```python
from build123d import *

# Parameters (mm, degrees)
SKETCH_R            = 2.95
PAD_DEPTH           = 1
SKETCH001_R         = 2.5
PAD001_DEPTH        = 7.7
FILLET_R            = 2.5
SKETCH002_W         = 0.7
SKETCH002_H         = 0.7
PAD002_DEPTH        = 0.5
SKETCH003_W         = 0.5
SKETCH003_H         = 0.5
PAD003_DEPTH        = 10.5
LINEARPATTERN_COUNT = 2
LINEARPATTERN_PITCH = 2.54


with BuildPart() as part:
    # Sketch → Pad (new body)
    with BuildSketch(Plane.XY):
        Circle(SKETCH_R)
    extrude(amount=PAD_DEPTH)

    # Sketch001 (on Face3 of Pad) → Pad001 (join)
    with BuildSketch(Plane.XY.offset(1)):
        Circle(SKETCH001_R)
    extrude(amount=PAD001_DEPTH)

    # Fillet
    fillet_edges = [part.edges().sort_by_distance(p)[0] for p in [
        (-2.5, 0, 8.7),
    ]]
    fillet(fillet_edges, radius=FILLET_R)

    # Sketch002 (on Face5 of Fillet) → Pad002 (join)
    with BuildSketch(Plane(origin=(0, 0, 0), x_dir=(1, 0, 0), z_dir=(0, 0, -1))):
        with Locations((-1.27, 0)):
            Rectangle(SKETCH002_W, SKETCH002_H)
    pad002 = extrude(amount=PAD002_DEPTH)

    # Sketch003 (on Face10 of Pad002) → Pad003 (join)
    with BuildSketch(Plane(origin=(0, 0, -0.5), x_dir=(1, 0, 0), z_dir=(0, 0, -1))):
        with Locations((-1.27, 0)):
            Rectangle(SKETCH003_W, SKETCH003_H)
    pad003 = extrude(amount=PAD003_DEPTH)

    # LinearPattern: Pad002, Pad003 ×2
    with Locations(*[(i * LINEARPATTERN_PITCH, 0, 0) for i in range(1, LINEARPATTERN_COUNT)]):
        add(pad002)
        add(pad003)


solid = part.part
```
Input: part model. Units: mm. Frame: model coordinates. A direction names the side the tool comes from. Coordinates: 2 decimals unless noted, no trailing zeros. Write each loop counter-clockwise with the first axis right and the second up, starting at its lowest first coordinate (ties: lowest second). Pieces come first, ordered by that corner, then holes. Notation, with made-up numbers: (84.5, -40) - (132.5, -40) arc R21 ccw to (132.5, -15) - close; hole circle Ø2 at (32.5, 83). An arc over 180 degrees is marked (long way). Put each result on its own line as item: value. Start each with the question number.
1) Reachability of faces 1 (the face through (-0.54, -2.44, 3.56)), 2 (the face through (-2.947, 0.13, 0.493)) from +Z, -Z, +X, -X, +Y, -Y: full face, straight path, thin tool, end or side. Return the list, or none.
2) Cut plane B-B (y = 0). Return the cut outline in (x, z), plus the area to 3 significant figures.
3) Contact query for flat-ended pins moving along their axis: pin 1 (0.6 mm diameter, centred on y = 0, z = -5.5, fed in from -X); pin 2 (1 mm diameter, centred on x = -0.5, y = -0.5, fed in from +Z); pin 3 (0.6 mm diameter, centred on x = 1.5, z = -3.5, fed in from +Y). Output: stop coordinate, or through.
4) Cut plane D-D (z = 3.5). Return the cut outline in (x, y), plus the area to 3 significant figures.
5) Ray query, L1, parallel to Y at x = 1.45, z = -6.5; L2, parallel to Z at x = -1.7, y = -1.9; L3, parallel to Y at x = 0.35, z = 5.5. Return the intervals inside material, ascending.
6) Cut plane C-C (x = 0). Return the cut outline in (y, z).
7) Cut plane A-A (z = -3.25). Return the cut outline in (x, y).
Resolved:
1. face 1: +Z
1. face 2: +Z, -Z
2. outline: (-2.95, 0) - (-1.62, 0) - (-1.62, -0.5) - (-1.52, -0.5) - (-1.52, -11) - (-1.02, -11) - (-1.02, -0.5) - (-0.92, -0.5) - (-0.92, 0) - (0.92, 0) - (0.92, -0.5) - (1.02, -0.5) - (1.02, -11) - (1.52, -11) - (1.52, -0.5) - (1.62, -0.5) - (1.62, 0) - (2.95, 0) - (2.95, 1) - (2.5, 1) - (2.5, 6.2) arc R2.5 ccw to (-2.5, 6.2) - (-2.5, 1) - (-2.95, 1) - close
2. area: 52.9 mm2
3. pin 1: stops at x = -1.52
3. pin 2: stops at z = 8.69
3. pin 3: stops at y = 0.25
4. outline: circle Ø5 at (0, 0)
4. area: 19.6 mm2
5. L1: y = -0.25 to 0.25
5. L2: z = 0 to 1
5. L3: y = -2.48 to 2.48
6. outline: (-2.95, 0) - (2.95, 0) - (2.95, 1) - (2.5, 1) - (2.5, 6.2) arc R2.5 ccw to (-2.5, 6.2) - (-2.5, 1) - (-2.95, 1) - close
7. outline: (-1.52, -0.25) - (-1.02, -0.25) - (-1.02, 0.25) - (-1.52, 0.25) - close; (1.02, -0.25) - (1.52, -0.25) - (1.52, 0.25) - (1.02, 0.25) - close
